Autodesk Inventor part; units mm, degrees
ref_plane "YZ Plane" through (0, 0, 0) normal (1, 0, 0) x (0, 1, 0)
ref_plane "XZ Plane" through (0, 0, 0) normal (0, 1, 0) x (-1, 0, 0)
ref_plane "XY Plane" through (0, 0, 0) normal (0, 0, 1) x (1, 0, 0)
sketch "Sketch1" plane through (0, 0, 0) normal (0, 0, 1) x (1, 0, 0)
  line L0 (19.05, -19.05) -> (-19.05, -19.05)
  line L1 (-19.05, -19.05) -> (-19.05, 19.05)
  line L2 (-19.05, 19.05) -> (19.05, 19.05)
  line L3 (19.05, 19.05) -> (19.05, -19.05)
  line L4 (19.05, -19.05) -> (-19.05, 19.05) construction
  line L5 (-19.05, -19.05) -> (19.05, 19.05) construction
  point P0 (0, 0)
  dimension "d0" = 38.1
  dimension "d1" = 38.1
extrude "Extrusion1" add sketch "Sketch1" along normal blind 6.35
sketch "Sketch2" plane through (0, 0, 6.35) normal (0, 0, 1) x (1, 0, 0)
  circle A0 centre (0, 0) radius 5.5309
  dimension "d4" = 11.0617
extrude "Extrusion2" add sketch "Sketch2" along normal blind 11.9634
sketch "Sketch3" plane through (0, 0, 18.3134) normal (0, 0, 1) x (1, 0, 0)
  circle A0 centre (0, 0) radius 2.9909
  line L0 (2.4956, 1.6485) -> (2.4956, -1.6485)
  dimension "d7" = 5.9817
  dimension "d8" = 5.4864
extrude "Extrusion3" cut sketch "Sketch3" against normal blind 11.9634 contours L0 A0 picked at (0.3599, 0.1211)
properties part number "Hub"
Design review of the part built by this model. Coordinates are the model's own, in mm. A direction names the side the tool comes from. Give positions to 0.01 mm unless a question says otherwise; leave off trailing zeros. Order: outer loops, then holes, each group sorted by start corner. A loop starts at its lowest first (then second) coordinate and runs counter-clockwise, first axis right, second up. Notation, with made-up numbers: (31.25, 67) - (59.25, 67) arc R21 ccw to (59.25, 89) - close; hole circle Ø9 at (67.5, 55.25). An arc over 180 degrees is marked (long way). Use a Markdown table: item, result. Add a question column.
(1) Add section D-D on z = 8.5. Give the boundary of the cut face in (x, y), then the cut area to 3 significant figures.
(2) Add section C-C on x = 4. Give the boundary of the cut face in (y, z), then the cut area to 3 significant figures.
(3) Clearance check with flat-ended pins moving along their axes: P1, Ø10, axis at x = -4.5, z = 12, coming from the +Y side; P2, Ø2.5, axis at x = -0.5, y = 0.5, coming from the +Z side; P3, Ø3.5, axis at y = -0.5, z = 12.5, coming from the -X side. State where each tip first meets the part, or that it passes through.
(4) Wall thickness on probe 1 along Y at (x, z) = (0, 9.75); probe 2 along Z at (x, y) = (0, 1); probe 3 along Y at (x, z) = (2, 17): over which ranges is each line inside the solid? List them lowest first. Write a range as [from, to].
(5) Mouldability with a two-part tool opening along Y and no side actions: class faces 3 (the face through (0, 0, 6.35)), 4 (the face through (19.05, 0, 3)), 5 (the face through (0, 19.05, 3)) as +Y half, -Y half, draft (parallel to the pull), parting line (faces both ways), or undercut.
(6) Add section B-B on y = 0. Give the boundary of the cut face in (x, z).
(7) Machinability: for faces 1 (the face through (-19.05, 0, 3)), 2 (the face through (2.496, 0, 12)), which of the approach directions +Z, -Z, +X, -X, +Y, -Y give a long, thin tool a straight path to every point of the face, cutting with its end or side? Answer none if there is none.
(8) Add section A-A on x = 0. Give the boundary of the cut face in (y, z).
Report:
| question | item | result |
|---|---|---|
| 1 | outline | circle Ø11.06 at (0, 0); hole (2.5, -1.65) - (2.5, 1.65) arc R2.99 ccw (long way) to start |
| 1 | area | 69.1 mm² |
| 2 | outline | (-19.05, 0) - (19.05, 0) - (19.05, 6.35) - (3.82, 6.35) - (3.82, 18.31) - (-3.82, 18.31) - (-3.82, 6.35) - (-19.05, 6.35) - close |
| 2 | area | 333 mm² |
| 3 | P1 | stops at y = 5.53 |
| 3 | P2 | stops at z = 6.35 |
| 3 | P3 | stops at x = -5.53 |
| 4 | probe 1 | y = [-5.53, -2.99], [2.99, 5.53] |
| 4 | probe 2 | z = [0, 6.35] |
| 4 | probe 3 | y = [-5.16, -2.22], [2.22, 5.16] |
| 5 | face 3 | undercut |
| 5 | face 4 | draft |
| 5 | face 5 | +Y half |
| 6 | outline | (-19.05, 0) - (19.05, 0) - (19.05, 6.35) - (5.53, 6.35) - (5.53, 18.31) - (2.5, 18.31) - (2.5, 6.35) - (-2.99, 6.35) - (-2.99, 18.31) - (-5.53, 18.31) - (-5.53, 6.35) - (-19.05, 6.35) - close |
| 7 | face 1 | +Z, -Z, -X, +Y, -Y |
| 7 | face 2 | +Z |
| 8 | outline | (-19.05, 0) - (19.05, 0) - (19.05, 6.35) - (5.53, 6.35) - (5.53, 18.31) - (2.99, 18.31) - (2.99, 6.35) - (-2.99, 6.35) - (-2.99, 18.31) - (-5.53, 18.31) - (-5.53, 6.35) - (-19.05, 6.35) - close |
